from build123d import *

# Parameters (mm, degrees)
CUT_EXTRUDE1_REACH      = 96.34
CUT_EXTRUDE1_END_RADIUS = 35
SKETCH2_R               = 3
CIRPATTERN1_COUNT       = 3


with BuildPart() as part:
    # Sketch1 → Revolve1 (revolve)
    with BuildSketch(Plane.XY, mode=Mode.PRIVATE) as revolve1_sk:
        Polygon((-40, 30), (0, 30), (0, 25), (-35, 25), (-35, 0), (-40, 0), align=None)
    revolve(revolve1_sk.sketch.rotate(Axis((0, -63.953488372, 0), (0, 1, 0)), 270), axis=Axis((0, -63.953488372, 0), (0, 1, 0)))

    # Cut-Extrude1: up to this cylinder (the profile starts outside it)
    cut_extrude1_end = Plane(origin=(0, 5, 0), z_dir=(0, -1, 0)) * Cylinder(CUT_EXTRUDE1_END_RADIUS, 263.68, mode=Mode.PRIVATE)
    # Sketch2 → Cut-Extrude1 (cut, up to the surface)
    with BuildSketch(Plane.XY.offset(40), mode=Mode.PRIVATE) as cut_extrude1_sk1:
        with Locations((0, 5)):
            Circle(SKETCH2_R)
    cut_extrude1_tool1 = extrude(cut_extrude1_sk1.sketch, amount=-CUT_EXTRUDE1_REACH, mode=Mode.PRIVATE) - cut_extrude1_end
    cut_extrude1 = cut_extrude1_tool1.solids().sort_by_distance((0, 5, 40))[0]
    add(cut_extrude1, mode=Mode.SUBTRACT)

    # CirPattern1: Cut-Extrude1 ×3 about axis
    cirpattern1_axis = Axis((0, -63.953488372, 0), (0, 1, 0))
    for i in range(1, CIRPATTERN1_COUNT):
        add(cut_extrude1.rotate(cirpattern1_axis, i * 360 / CIRPATTERN1_COUNT), mode=Mode.SUBTRACT)


solid = part.part
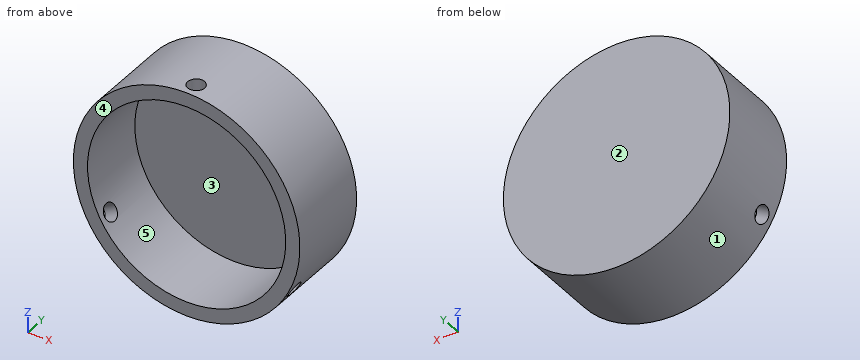
Can you work these out from the model? Positions are in its coordinate system, mm. Face numbers are marked on the shaded views. A direction names the side the tool comes from. Give positions to 0.01 mm unless a question says otherwise; leave off trailing zeros. Order: outer loops, then holes, each group sorted by start corner. A loop starts at its lowest first (then second) coordinate and runs counter-clockwise, first axis right, second up. Notation, with made-up numbers: (24, -37.5) - (81, -37.5) arc R10 ccw to (81, -24.5) - close; hole circle Ø10 at (63.5, -7). An arc over 180 degrees is marked (long way). Write each question's results on one line, items separated by ' | '.
1) Suppose I cut it at A-A, the plane x = 0. Write out the boundary of the cut face in (y, z), then the cut area to 3 significant figures.
Final values:
outline: (0, -40) - (30, -40) - (30, 40) - (8, 40) - (8, 35) - (25, 35) - (25, -35) - (0, -35) - close; (0, 35) - (2, 35) - (2, 40) - (0, 40) - close | area: 620 mm^2
2) Suppose I cut it at C-C, the plane z = 0. Write out the boundary of the cut face in (x, y).
Final values:
outline: (-40, 0) - (-35, 0) - (-35, 25) - (35, 25) - (35, 0) - (40, 0) - (40, 30) - (-40, 30) - close
3) I'm going to push flat-ended pins straight in: pin 1 Ø4 at (x, y) = (31.5, 24) entering from -Z; pin 2 Ø1 at (x, y) = (11, 11.5) entering from -Z; pin 3 Ø3 at (x, y) = (30.5, 13.5) entering from +Z. Where does each tip first touch, or does it pass through?
Final values:
pin 1: stops at z = -27.01 | pin 2: stops at z = -38.6 | pin 3: stops at z = 27.55
4) Suppose I cut it at B-B, the plane y = 5. Write out the boundary of the cut face in (x, z).
Final values:
outline: (-36.04, -17.35) - (-31.7, -14.84) arc R35 cw to (-3, 34.87) - (-3, 39.89) arc R40 ccw to start; (-33.04, -22.54) arc R40 ccw to (33.04, -22.54) - (28.7, -20.03) arc R35 cw to (-28.7, -20.03) - close; (3, 34.87) arc R35 cw to (31.7, -14.84) - (36.04, -17.35) arc R40 ccw to (3, 39.89) - close
5) If we mould it in two halves opening along Z, with no side actions, what happens to the marked faces 1, 2 and 3? For each: pulls with the +Z half, pulls with the -Z half, needs draft (parallel to the pull), parting line crosses it, or undercut.
Final values:
face 1: parting line crosses it | face 2: needs draft | face 3: undercut
6) On a 3-axis mill with a long thin cutter (end or side, diameter ignored), from which of +Z, -Z, +X, -X, +Y, -Y can I reach the whole of each face in a straight line? I mean the marked faces 4 and 5. Say none if no direction works.
Final values:
face 4: +Z, -Z, +X, -X, -Y | face 5: -Y
7) Suppose I cut it at D-D, the plane y = 21.5. Write out the boundary of the cut face in (x, z).
Final values:
outline: circle Ø80 at (0, 0); hole circle Ø70 at (0, 0)
8) Please list where these lines run through material, in increasing order: line 1 along Z through (x, y) = (0.5, 2); line 2 along X through (y, z) = (18, 1); line 3 along Y through (x, z) = (0, 38). Write a range as [from, to].
Final values:
line 1: z = [-40, -35], [35, 40] | line 2: x = [-39.99, -34.99], [34.99, 39.99] | line 3: y = [0, 2], [8, 30]
